from build123d import *

# Parameters (mm, degrees)
SKETCH1_R           = 28
BOSS_EXTRUDE1_DEPTH = 4
SKETCH2_R           = 6
BOSS_EXTRUDE2_DEPTH = 4
SKETCH4_R           = 1.197375231
CUT_EXTRUDE2_DEPTH  = 46.683525867
SKETCH5_R           = 12.5
CUT_EXTRUDE3_DEPTH  = 46.683525867
BOSS_EXTRUDE3_START = 8
SKETCH6_R           = 15.7
SKETCH6_R_2         = 12.5
BOSS_EXTRUDE3_DEPTH = 8
SKETCH7_W           = 30.4
SKETCH7_H           = 10.4
BOSS_EXTRUDE4_DEPTH = 4
SKETCH8_W           = 30.4
SKETCH8_H           = 4
BOSS_EXTRUDE5_DEPTH = 12
FILLET1_R           = 4
FILLET2_R           = 1.6
SKETCH9_R           = 1.55
CUT_EXTRUDE4_DEPTH  = 5


with BuildPart() as part:
    # Sketch1 → Boss-Extrude1 (new body)
    with BuildSketch(Plane(origin=(0, 0, 0), x_dir=(1, 0, 0), z_dir=(0, 1, 0))):
        with Locations(Location((0, 0, 0), (0, 0, 270))):
            Circle(SKETCH1_R)
    extrude(amount=BOSS_EXTRUDE1_DEPTH)

    # Sketch2 → Boss-Extrude2 (add)
    with BuildSketch(Plane(origin=(0, 4, 0), x_dir=(1, 0, 0), z_dir=(0, 1, 0))):
        with Locations((28, 0)):
            Circle(SKETCH2_R)
        with Locations((-14, -24.248711306)):
            Circle(SKETCH2_R)
        with Locations((-14, 24.248711306)):
            Circle(SKETCH2_R)
    extrude(amount=-BOSS_EXTRUDE2_DEPTH)

    # Sketch4 → Cut-Extrude2 (cut, through all)
    with BuildSketch(Plane(origin=(0, 4, 0), x_dir=(1, 0, 0), z_dir=(0, 1, 0))):
        with Locations(Location((28.8, 0, 0), (0, 0, 270))):
            Circle(SKETCH4_R)
        with Locations(Location((-14.4, -24.941531629, 0), (0, 0, 270))):
            Circle(SKETCH4_R)
        with Locations(Location((-14.4, 24.941531629, 0), (0, 0, 270))):
            Circle(SKETCH4_R)
    extrude(amount=-CUT_EXTRUDE2_DEPTH, mode=Mode.SUBTRACT)

    # Sketch5 → Cut-Extrude3 (cut, through all)
    with BuildSketch(Plane(origin=(0, 4, 0), x_dir=(1, 0, 0), z_dir=(0, 1, 0))):
        with Locations(Location((0, 0, 0), (0, 0, 270))):
            Circle(SKETCH5_R)
    extrude(amount=-CUT_EXTRUDE3_DEPTH, mode=Mode.SUBTRACT)

    # Sketch6 → Boss-Extrude3 (add)
    with BuildSketch(Plane(origin=(0, 4, 0), x_dir=(1, 0, 0), z_dir=(0, 1, 0)).offset(BOSS_EXTRUDE3_START)):
        with Locations(Location((0, 0, 0), (0, 0, 270))):
            Circle(SKETCH6_R)
        with Locations(Location((0, 0, 0), (0, 0, 270))):
            Circle(SKETCH6_R_2, mode=Mode.SUBTRACT)
    extrude(amount=-BOSS_EXTRUDE3_DEPTH)

    # Sketch7 → Boss-Extrude4 (add)
    with BuildSketch(Plane(origin=(0, 4, 0), x_dir=(1, 0, 0), z_dir=(0, 1, 0))):
        with Locations((3.65, -25.448711306)):
            Rectangle(SKETCH7_W, SKETCH7_H)
    extrude(amount=-BOSS_EXTRUDE4_DEPTH)

    # Sketch8 → Boss-Extrude5 (add)
    with BuildSketch(Plane(origin=(0, 4, 0), x_dir=(1, 0, 0), z_dir=(0, 1, 0))):
        with Locations((3.65, -28.648711306)):
            Rectangle(SKETCH8_W, SKETCH8_H)
    extrude(amount=BOSS_EXTRUDE5_DEPTH)

    # Fillet1
    fillet1_edges = [part.edges().sort_by_distance(p)[0] for p in [
        (3.65, 4, 26.648711306),
    ]]
    fillet(fillet1_edges, radius=FILLET1_R)

    # Fillet2
    fillet2_edges = [part.edges().sort_by_distance(p)[0] for p in [
        (18.85, 16, 28.648711306),
        (3.65, 16, 26.648711306),
        (-11.55, 16, 28.648711306),
        (3.65, 16, 30.648711306),
    ]]
    fillet(fillet2_edges, radius=FILLET2_R)

    # Sketch9 → Cut-Extrude4 (cut)
    with BuildSketch(Plane.XY.offset(30.648711306)):
        with Locations((-3.55, 9.6)):
            Circle(SKETCH9_R)
        with Locations((10.85, 9.6)):
            Circle(SKETCH9_R)
    extrude(amount=-CUT_EXTRUDE4_DEPTH, mode=Mode.SUBTRACT)


solid = part.part
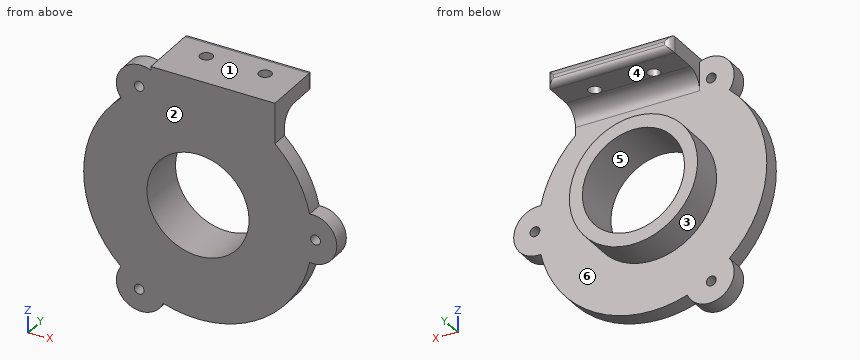
Could you check a few things on this model? Use its own coordinates, in mm. Face numbers are marked on the shaded views. A direction names the side the tool comes from. Round coordinates to 2 decimals unless told otherwise and drop trailing zeros. Loops run counter-clockwise (first coordinate to the right, second up) from the corner with the lowest first, then second, coordinate; pieces in that order, holes last. Notation, with made-up numbers: (50.25, 7.25) -> (62.25, 7.25) arc R12 ccw to (62.25, 24.25) -> close; hole circle Ø8 at (47, -21.5). An arc over 180 degrees is marked (long way). Use CSV: the item, a comma, the result in double quotes.
(1) Suppose I cut it at D-D on z = 11.5. Write out the boundary of the cut face in (x, y).
Return value:
outline,"(-25.53, 0) -> (-4.9, 0) -> (-4.9, 12) -> (-10.69, 12) -> (-10.69, 4) -> (-25.53, 4) -> close; (4.9, 0) -> (25.53, 0) -> (25.53, 4) -> (10.69, 4) -> (10.69, 12) -> (4.9, 12) -> close"
(2) Will these pins go through, and if not, where does the flat tip stop? pin 1 Ø6.5 at (y, z) = (10, 28.5) entering from -X; pin 2 Ø1.4 at (x, z) = (-14.4, 24.94) entering from +Y; pin 3 Ø5 at (y, z) = (13.5, -7) entering from +X; pin 4 Ø5 at (x, z) = (21.5, -6.5) entering from +Y.
Return value:
pin 1,"stops at x = -11.55"
pin 2,"passes through"
pin 3,"stops at x = 14.88"
pin 4,"stops at y = 4"
(3) Suppose I cut it at A-A on y = 9.6. Write out the boundary of the cut face in (x, z).
Return value:
outline,"circle Ø31.4 at (0, 0); (-11.55, 26.65) -> (-5.1, 26.65) -> (-5.1, 30.65) -> (-11.55, 30.65) -> close; (-2, 26.65) -> (9.3, 26.65) -> (9.3, 30.65) -> (-2, 30.65) -> close; (12.4, 26.65) -> (18.85, 26.65) -> (18.85, 30.65) -> (12.4, 30.65) -> close; hole circle Ø25 at (0, 0)"
(4) Suppose I cut it at B-B on x = 0. Write out the boundary of the cut face in (y, z).
Return value:
outline,"(0, -28) -> (4, -28) -> (4, -15.7) -> (12, -15.7) -> (12, -12.5) -> (0, -12.5) -> close; (0, 12.5) -> (12, 12.5) -> (12, 15.7) -> (4, 15.7) -> (4, 22.65) arc R4 cw to (8, 26.65) -> (14.4, 26.65) arc R1.6 ccw to (16, 28.25) -> (16, 29.05) arc R1.6 ccw to (14.4, 30.65) -> (0, 30.65) -> close"
(5) If I drill on probe 1 along Z at (x, y) = (-19.5, 3); probe 2 along Z at (x, y) = (1, 11); probe 3 along Y at (x, z) = (10.85, 28.3), over which ranges is the centre line in solid material (lowest first)? Write a range as [from, to].
Return value:
probe 1,"z = [-26.65, -21.85], [-20.09, 20.09], [21.85, 26.65]"
probe 2,"z = [-15.67, -12.46], [12.46, 15.67], [26.65, 30.65]"
probe 3,"y = [0, 8.05], [11.15, 16]"
(6) For the marked faces 4, 5 and 6, which set-ups out of +Z, -Z, +X, -X, +Y, -Y let a thin tool reach every point of the face, with its end or its side?
Return value:
face 4,"+X, -X, +Y"
face 5,"+Y, -Y"
face 6,"+Y"
(7) Suppose I cut it at C-C on x = 10.85. Write out the boundary of the cut face in (y, z).
Return value:
outline,"(0, -25.81) -> (4, -25.81) -> (4, -11.35) -> (12, -11.35) -> (12, -6.21) -> (0, -6.21) -> close; (0, 6.21) -> (12, 6.21) -> (12, 11.35) -> (4, 11.35) -> (4, 22.65) arc R4 cw to (8, 26.65) -> (8.05, 26.65) -> (8.05, 30.65) -> (0, 30.65) -> close; (11.15, 26.65) -> (14.4, 26.65) arc R1.6 ccw to (16, 28.25) -> (16, 29.05) arc R1.6 ccw to (14.4, 30.65) -> (11.15, 30.65) -> close"
(8) If we mould it in two halves opening along Z, with no side actions, what happens to the marked faces 1, 2 and 3? For each: +Z half, -Z half, draft (parallel to the pull), parting line (faces both ways), or undercut.
Return value:
face 1,"+Z half"
face 2,"draft"
face 3,"undercut"
